Build history of the part. All positions in model axes, mm. A direction names the side the tool comes from. Coordinates: 2 decimals unless noted, no trailing zeros. Loops run counter-clockwise (first coordinate to the right, second up) from the corner with the lowest first, then second, coordinate; pieces in that order, holes last.
Item 1: Cut at C-C (y = 2.25). List the corners of the cut face in (x, z) (3 decimals).
Item 2: Cut at D-D (z = 5.75). List the corners of the cut face in (x, y), and give its area (3 significant figures).
Item 3: Cut at B-B (x = 1.5). List the corners of the cut face in (y, z).
Item 4: Cut at A-A (z = 0). List the corners of the cut face in (x, y) (3 decimals).
Item 5: 3-axis set-ups, long thin cutter, end or side, ignore diameter. For faces 1 (the face through (6, -6.35, 0)), 2 (the face through (-14.09, -3.1, 0.69)): which of +Z, -Z, +X, -X, +Y, -Y reach the whole face in a straight line?
Item 6: Drill centre lines: line 1 along X through (y, z) = (-3, -5.25); line 2 along Z through (x, y) = (-9.5, -2.5); line 3 along Y through (x, z) = (1, -4.5). Where is each one in solid material? Low to high.
Item 7: Mould opens along X. For faces 3 (the face through (11.43, 0, 0)), 4 (the face through (0, 3, -2)), 5 (the face through (5.635, 3.219, 5.474)) say: released by +X, released by -X, zero draft, split by the parting line, or undercut.
Item 8: Flat gauge pins, fed straight in: pin 1 (5 mm diameter, centred on x = -22, y = 3, fed in from +Z); pin 2 (8 mm diameter, centred on x = -19, z = 6, fed in from -Y); pin 3 (5 mm diameter, centred on x = 4.5, z = 5.5, fed in from +Y); pin 4 (2 mm diameter, centred on x = -24, y = 3, fed in from -Z). Where does each tip first touch, or does it go through?
from build123d import *

# Parameters (mm, degrees)
SKETCH1_R           = 3.175
BOSS_EXTRUDE1_DEPTH = 11.43
SKETCH1_3_R         = 3.175
BOSS_EXTRUDE2_DEPTH = 28.575


with BuildPart() as part:
    # Sketch1 → Boss-Extrude1 (new body)
    # profile 1 of 2: a face of its own
    with BuildSketch(Plane(origin=(0, 0, 0), x_dir=(0, 0, -1), z_dir=(1, 0, 0))):
        Polygon((3.666174209, -6.35), (7.332348419, 0), (3.666174209, 6.35), (-3.666174209, 6.35), (-7.332348419, 0), (-3.666174209, -6.35), align=None)
        Circle(SKETCH1_R, mode=Mode.SUBTRACT)
    # profile 2 of 2: a face of its own
    with BuildSketch(Plane(origin=(0, 0, 0), x_dir=(0, 0, -1), z_dir=(1, 0, 0))):
        Circle(SKETCH1_R)
    extrude(amount=BOSS_EXTRUDE1_DEPTH)

    # Sketch1<3> → Boss-Extrude2 (add)
    with BuildSketch(Plane(origin=(0, 0, 0), x_dir=(0, 0, -1), z_dir=(1, 0, 0))):
        Circle(SKETCH1_3_R)
    extrude(amount=-BOSS_EXTRUDE2_DEPTH)


solid = part.part
Filled sheet:
1. outline: (-28.575, -2.24) - (0, -2.24) - (0, -6.033) - (11.43, -6.033) - (11.43, 6.033) - (0, 6.033) - (0, 2.24) - (-28.575, 2.24) - close
2. outline: (0, -2.74) - (11.43, -2.74) - (11.43, 2.74) - (0, 2.74) - close
2. area: 62.7 mm2
3. outline: (-6.35, -3.67) - (0, -7.33) - (6.35, -3.67) - (6.35, 3.67) - (0, 7.33) - (-6.35, 3.67) - close
4. outline: (-28.575, -3.175) - (0, -3.175) - (0, -6.35) - (11.43, -6.35) - (11.43, 6.35) - (0, 6.35) - (0, 3.175) - (-28.575, 3.175) - close
5. face 1: +Z, -Z, +X, -X, -Y
5. face 2: -X
6. line 1: x = 0 to 11.43
6. line 2: z = -1.96 to 1.96
6. line 3: y = -4.91 to 4.91
7. face 3: released by +X
7. face 4: released by -X
7. face 5: zero draft
8. pin 1: stops at z = 3.14
8. pin 2: stops at y = -2.47
8. pin 3: stops at y = 6.35
8. pin 4: stops at z = -2.47
